Source: CAD feature listing. Evaluate the final solid. Frame: model axes, mm. Face numbers are marked on the shaded views. Round coordinates to 2 decimals unless told otherwise and drop trailing zeros. Loops run counter-clockwise (first coordinate to the right, second up) from the corner with the lowest first, then second, coordinate; pieces in that order, holes last. Notation, with made-up numbers: (10.5, -21.5) -> (65.5, -21.5) arc R9 ccw to (65.5, -12.5) -> close; hole circle Ø10 at (5, 83.25). An arc over 180 degrees is marked (long way). Put each result on its own line as item: value. Start each with the question number.
1. Cut plane C-C (y = -62). Return the cut outline in (x, z) (3 decimals).
2. Draft query along X for the marked faces 1, 2 and 3. Return one class per face: pulls with the +X half, pulls with the -X half, needs draft (parallel to the pull), parting line crosses it, or undercut.
3. Cut plane B-B (z = -58). Return the cut outline in (x, y) (3 decimals), then the cut area to 3 significant figures.
4. Cut plane D-D (y = -19.5). Return the cut outline in (x, z) (3 decimals).
5. Material intervals for L1, parallel to Z at x = -4.5, y = -36 (3 decimals); L2, parallel to X at y = -53, z = -3; L3, parallel to Y at x = 5.5, z = -4.5, sorted ascending.
6. Contact query for flat-ended pins moving along their axis: pin 1 (2.5 mm diameter, centred on x = 7, y = -1, fed in from -Z) (3 decimals); pin 2 (5 mm diameter, centred on x = -4, z = -47.5, fed in from -Y); pin 3 (4 mm diameter, centred on x = 0.5, y = -23, fed in from -Z). Output: stop coordinate, or through.
```python
from build123d import *

# Parameters (mm, degrees)
SKETCH5_W           = 12.880016042
SKETCH5_H           = 15.834691301
CUT_EXTRUDE2_DEPTH  = 7.62
CUT_EXTRUDE6_REACH  = 62
SKETCH11_W          = 3.175
SKETCH11_H          = 3.175
BOSS_EXTRUDE1_DEPTH = 6.35
CUT_EXTRUDE4_DEPTH  = 3.175
CUT_EXTRUDE7_DEPTH  = 40.64
BOSS_EXTRUDE3_DEPTH = 12.7
SKETCH19_W          = 21.319602533
SKETCH19_H          = 36.10119369
CUT_EXTRUDE10_DEPTH = 13.7
SKETCH15_W          = 6.35
SKETCH15_H          = 3.175
BOSS_EXTRUDE2_DEPTH = 1.5875
SKETCH20_W          = 6.35
SKETCH20_H          = 4
CUT_EXTRUDE11_DEPTH = 108.95


with BuildPart() as part:
    # Sketch2 → Revolve1 (revolve)
    with BuildSketch(Plane(origin=(0, 0, 0), x_dir=(0, 0, -1), z_dir=(1, 0, 0))):
        Polygon((0, -50.8), (-29.999999944, 0), (0, 0), align=None)
    revolve(axis=Axis((0, 0, 0), (0, -1, 0)))

    # Sketch4 → Cut-Revolve1 (revolve, cut)
    with BuildSketch(Plane(origin=(0, 0, 0), x_dir=(0, 0, -1), z_dir=(1, 0, 0))):
        Polygon((0, -45.72), (-24.919999944, 0), (0, 0), align=None)
    revolve(axis=Axis((0, 16.11457811, 0), (0, -1, 0)), mode=Mode.SUBTRACT)

    # Sketch5 → Cut-Extrude2 (cut, symmetric)
    with BuildSketch(Plane(origin=(0, 0, 0), x_dir=(0, 0, -1), z_dir=(1, 0, 0))):
        with Locations((0, -47.812265381)):
            Rectangle(SKETCH5_W, SKETCH5_H)
    extrude(amount=CUT_EXTRUDE2_DEPTH, both=True, mode=Mode.SUBTRACT)

    # Sketch11 → Cut-Extrude6 (cut, up to next)
    with BuildSketch(Plane.XY.offset(29.999999944), mode=Mode.PRIVATE) as cut_extrude6_sk1:
        with Locations((4.7625, -1.5875)):
            Rectangle(SKETCH11_W, SKETCH11_H)
    cut_extrude6_tool1 = extrude(cut_extrude6_sk1.sketch, amount=-CUT_EXTRUDE6_REACH, mode=Mode.PRIVATE) & part.part
    add(cut_extrude6_tool1.solids().sort_by_distance((4.7625, -1.5875, 30))[0], mode=Mode.SUBTRACT)
    # Sketch11 → Cut-Extrude6 (cut, up to next)
    with BuildSketch(Plane.XY.offset(29.999999944), mode=Mode.PRIVATE) as cut_extrude6_sk2:
        with Locations((-4.7625, -1.5875)):
            Rectangle(SKETCH11_W, SKETCH11_H)
    cut_extrude6_tool2 = extrude(cut_extrude6_sk2.sketch, amount=-CUT_EXTRUDE6_REACH, mode=Mode.PRIVATE) & part.part
    add(cut_extrude6_tool2.solids().sort_by_distance((-4.7625, -1.5875, 30))[0], mode=Mode.SUBTRACT)

    # Sketch6 → Boss-Extrude1 (add, symmetric)
    with BuildSketch(Plane(origin=(0, 0, 0), x_dir=(0, 0, -1), z_dir=(1, 0, 0))):
        with BuildLine():
            Line((0, -39.89491973), (-7.374618631, -39.89491973))
            Line((-7.374618631, -39.89491973), (11.56279342, -71.962270863))
            ThreePointArc((11.56279342, -71.962270863), (29.890602823, -92.707185326), (54.61, -105.165575141))
            ThreePointArc((54.61, -105.165575141), (64.513552335, -107.250553005), (74.61, -107.95))
            Line((74.61, -107.95), (77.785, -107.95))
            Line((77.785, -107.95), (77.785, -98.425))
            Line((77.785, -98.425), (74.61, -98.425))
            Line((74.61, -98.425), (74.61, -101.6))
            ThreePointArc((74.61, -101.6), (41.460280796, -92.804941633), (17.03053379, -68.733290336))
            Line((17.03053379, -68.733290336), (0, -39.89491973))
        make_face()
        Polygon((-30.934610553, 0), (-7.374618631, -39.89491973), (0, -39.89491973), (-23.559991923, 0), align=None)
    extrude(amount=BOSS_EXTRUDE1_DEPTH, both=True)

    # Sketch7 → Cut-Extrude4 (cut)
    with BuildSketch(Plane(origin=(0, 0, 0), x_dir=(0, 0, -1), z_dir=(1, 0, 0))):
        with BuildLine():
            Line((-3.175, -39.89491973), (14.676503495, -70.123465704))
            ThreePointArc((14.676503495, -70.123465704), (36.599939349, -93.039017482), (66.414189392, -103.849662572))
            ThreePointArc((66.414189392, -103.849662572), (70.51080038, -104.32379518), (74.61, -104.775))
            Line((74.61, -104.775), (74.61, -101.6))
            ThreePointArc((74.61, -101.6), (59.345071166, -99.83437787), (44.886242604, -94.630749287))
            ThreePointArc((44.886242604, -94.630749287), (29.078331812, -83.704237641), (17.03053379, -68.733290336))
            Line((17.03053379, -68.733290336), (-23.559991923, 0))
            Line((-23.559991923, 0), (-26.734991923, 0))
            Line((-26.734991923, 0), (-3.175, -39.89491973))
        make_face()
    cut_extrude4 = extrude(amount=-CUT_EXTRUDE4_DEPTH, mode=Mode.SUBTRACT)

    # Mirror1: Cut-Extrude4 across plane
    add(cut_extrude4.mirror(Plane(origin=(0, 0, 0), x_dir=(0, 0, 1), z_dir=(1, 0, 0))), mode=Mode.SUBTRACT)

    # Sketch9 → Cut-Revolve2 (revolve, cut)
    with BuildSketch(Plane(origin=(0, 0, 0), x_dir=(0, 0, -1), z_dir=(1, 0, 0))):
        Polygon((0, 0), (-24.9199908, 0), (-0.536470716, -39.89491973), (0, -39.89491973), align=None)
    revolve(axis=Axis((0, 16.11457811, 0), (0, -1, 0)), mode=Mode.SUBTRACT)

    # Sketch12 → Cut-Extrude7 (cut, symmetric)
    with BuildSketch(Plane.ZY):
        Polygon((30, 0), (-61.025869449, 0), (-61.025869449, -39.89491973), (-6.440008021, -39.89491973), (6.44000802, -39.89491973), (27.945214206, -3.175), align=None)
    extrude(amount=CUT_EXTRUDE7_DEPTH, both=True, mode=Mode.SUBTRACT)

    # Sketch18 → Boss-Extrude3 (add)
    with BuildSketch(Plane.ZY.offset(6.35)):
        with BuildLine():
            Line((6.44000802, -39.89491973), (6.44000802, 0))
            Line((6.44000802, 0), (9.61500802, 0))
            Line((9.61500802, 0), (9.61500802, -34.473639686))
            Line((9.61500802, -34.473639686), (9.61500802, -36.10119369))
            ThreePointArc((9.61500802, -36.10119369), (8.57844205, -39.89491973), (5.756782033, -42.634456374))
            Line((5.756782033, -42.634456374), (6.44000802, -41.477527034))
            Line((6.44000802, -41.477527034), (6.44000802, -39.89491973))
        make_face()
    extrude(amount=-BOSS_EXTRUDE3_DEPTH)

    # Sketch19 → Cut-Extrude10 (cut, through all)
    with BuildSketch(Plane.ZY.offset(6.35)):
        with Locations((20.274809287, -18.050596845)):
            Rectangle(SKETCH19_W, SKETCH19_H)
    extrude(amount=-CUT_EXTRUDE10_DEPTH, mode=Mode.SUBTRACT)

    # Sketch15 → Boss-Extrude2 (add, symmetric)
    with BuildSketch(Plane.ZY.offset(6.35)):
        with Locations((6.44000802, -1.5875)):
            Rectangle(SKETCH15_W, SKETCH15_H)
    boss_extrude2 = extrude(amount=BOSS_EXTRUDE2_DEPTH, both=True)

    # Mirror2: Boss-Extrude2 across plane
    add(boss_extrude2.mirror(Plane(origin=(0, 0, 0), x_dir=(0, 0, 1), z_dir=(1, 0, 0))))

    # Sketch20 → Cut-Extrude11 (cut, through all)
    with BuildSketch(Plane(origin=(0, 0, 0), x_dir=(1, 0, 0), z_dir=(0, 1, 0))):
        with Locations((0, 72.61)):
            Rectangle(SKETCH20_W, SKETCH20_H)
    extrude(amount=-CUT_EXTRUDE11_DEPTH, mode=Mode.SUBTRACT)


solid = part.part
```
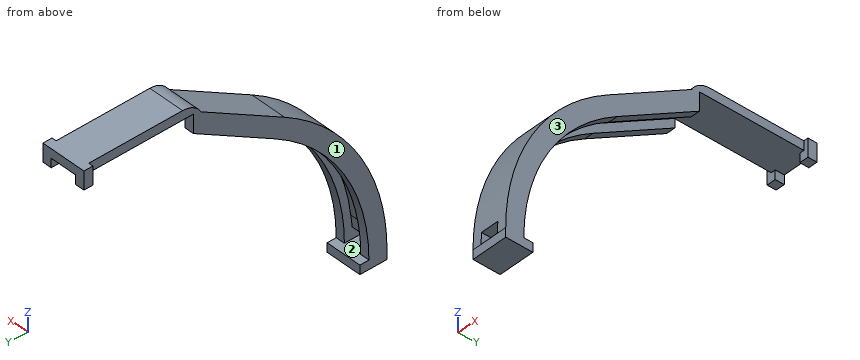
Solution:
1. outline: (-6.35, -13.054) -> (-3.175, -13.054) -> (-3.175, -9.879) -> (3.175, -9.879) -> (3.175, -13.054) -> (6.35, -13.054) -> (6.35, -5.68) -> (-6.35, -5.68) -> close
2. face 1: pulls with the -X half
2. face 2: undercut
2. face 3: pulls with the +X half
3. outline: (-6.35, -106.041) -> (6.35, -106.041) -> (6.35, -99.504) -> (3.175, -99.504) -> (3.175, -102.323) -> (-3.175, -102.323) -> (-3.175, -99.504) -> (-6.35, -99.504) -> close
3. area: 65.1 mm^2
4. outline: (-6.35, 6.44) -> (6.35, 6.44) -> (6.35, 9.615) -> (-6.35, 9.615) -> close
5. L1: z = 6.44 to 9.615
5. L2: x = -6.35 to 6.35
5. L3: y = -60 to -47.51
6. pin 1: stops at z = 3.265
6. pin 2: stops at y = -103.69
6. pin 3: stops at z = 6.44
